Verification items for the finished model (mm, model axes). Round coordinates to 2 decimals unless told otherwise and drop trailing zeros. Order: outer loops, then holes, each group sorted by start corner. A loop starts at its lowest first (then second) coordinate and runs counter-clockwise, first axis right, second up. Notation, with made-up numbers: (87.5, 80) -> (135.5, 80) arc R12 ccw to (135.5, 85) -> close; hole circle Ø7 at (66, 18.5). An arc over 180 degrees is marked (long way). Put each result on its own line as item: value.
from build123d import *

# Parameters (mm, degrees)
SKETCH_1_W          = 100
SKETCH_1_H          = 20
EXTRUDE_1_DEPTH     = 5.5
SKETCH_2_R          = 1.6
SKETCH_2_R_2        = 1.05
SKETCH_2_W          = 22.5
SKETCH_2_H          = 12.2
CUT_EXTRUDE_1_DEPTH = 52.285962992


with BuildPart() as part:
    # ｽｹｯﾁ1 → ﾎﾞｽ - 押し出し1 (new body)
    with BuildSketch(Plane.XY):
        Rectangle(SKETCH_1_W, SKETCH_1_H)
    extrude(amount=EXTRUDE_1_DEPTH)

    # ｽｹｯﾁ2 → ｶｯﾄ - 押し出し1 (cut, through all)
    with BuildSketch(Plane.XY.offset(5.5)):
        with Locations((-42.5, 0)):
            Circle(SKETCH_2_R)
        with Locations((42.5, 0)):
            Circle(SKETCH_2_R)
        with Locations((-8.75, 0)):
            Circle(SKETCH_2_R_2)
        with Locations((19.05, 0)):
            Circle(SKETCH_2_R_2)
        with Locations((5.15, 0)):
            Rectangle(SKETCH_2_W, SKETCH_2_H)
    extrude(amount=-CUT_EXTRUDE_1_DEPTH, mode=Mode.SUBTRACT)


solid = part.part
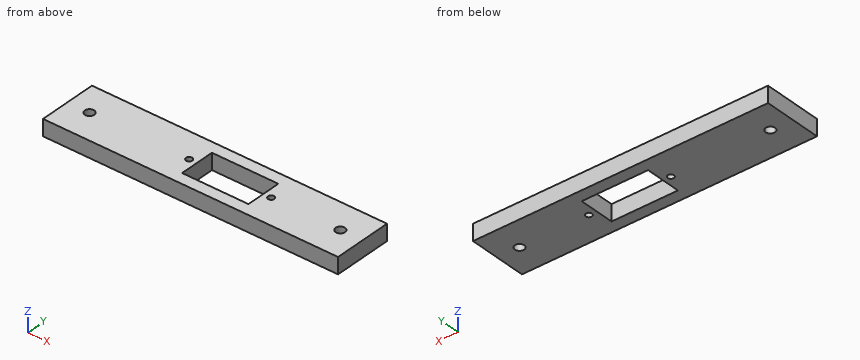
Item 1: Section check B-B on y = 0. Record the boundary of the cut face in (x, z), then the cut area to 3 significant figures.
Check sheet entries:
outline: (-50, 0) -> (-44.1, 0) -> (-44.1, 5.5) -> (-50, 5.5) -> close; (-40.9, 0) -> (-9.8, 0) -> (-9.8, 5.5) -> (-40.9, 5.5) -> close; (-7.7, 0) -> (-6.1, 0) -> (-6.1, 5.5) -> (-7.7, 5.5) -> close; (16.4, 0) -> (18, 0) -> (18, 5.5) -> (16.4, 5.5) -> close; (20.1, 0) -> (40.9, 0) -> (40.9, 5.5) -> (20.1, 5.5) -> close; (44.1, 0) -> (50, 0) -> (50, 5.5) -> (44.1, 5.5) -> close
area: 368 mm^2
Item 2: Section check D-D on x = -8.75. Record the boundary of the cut face in (y, z), then the cut area to 4 significant figures.
Check sheet entries:
outline: (-10, 0) -> (-1.05, 0) -> (-1.05, 5.5) -> (-10, 5.5) -> close; (1.05, 0) -> (10, 0) -> (10, 5.5) -> (1.05, 5.5) -> close
area: 98.45 mm^2
Item 3: Section check C-C on z = 4.55. Record the boundary of the cut face in (x, y), then the cut area to 3 significant figures.
Check sheet entries:
outline: (-50, -10) -> (50, -10) -> (50, 10) -> (-50, 10) -> close; hole circle Ø3.2 at (-42.5, 0); hole circle Ø2.1 at (-8.75, 0); hole (-6.1, -6.1) -> (16.4, -6.1) -> (16.4, 6.1) -> (-6.1, 6.1) -> close; hole circle Ø2.1 at (19.05, 0); hole circle Ø3.2 at (42.5, 0)
area: 1,700 mm^2
Item 4: Gauge pin test, flat end, axial feed: pin 1 Ø2.5 at (x, y) = (19.05, 0) entering from +Z. Record the tip position at first contact, or that the pin passes through.
Check sheet entries:
pin 1: stops at z = 5.5
Item 5: Material ranges on L1, parallel to Y at x = -42.5, z = 4.4; L2, parallel to Y at x = -6, z = 2.2; L3, parallel to X at y = 5.25, z = 1.7, recorded low to high. Write a range as [from, to].
Check sheet entries:
L1: y = [-10, -1.6], [1.6, 10]
L2: y = [-10, -6.1], [6.1, 10]
L3: x = [-50, -6.1], [16.4, 50]
Item 6: Section check A-A on x = 42.5. Record the boundary of the cut face in (y, z), then the cut area to 3 significant figures.
Check sheet entries:
outline: (-10, 0) -> (-1.6, 0) -> (-1.6, 5.5) -> (-10, 5.5) -> close; (1.6, 0) -> (10, 0) -> (10, 5.5) -> (1.6, 5.5) -> close
area: 92.4 mm^2
